Build history of the part. All positions in model axes, mm. Face numbers are marked on the shaded views. Give positions to 0.01 mm unless a question says otherwise; leave off trailing zeros. Order: outer loops, then holes, each group sorted by start corner. A loop starts at its lowest first (then second) coordinate and runs counter-clockwise, first axis right, second up. Notation, with made-up numbers: (62, 73) - (76, 73) arc R13 ccw to (76, 77) - close; hole circle Ø2 at (25, 48.5). An arc over 180 degrees is marked (long way). One line per item, written item: value.
```python
from build123d import *

# Parameters (mm, degrees)
SKETCH1_R                  = 12.5
SKETCH1_R_2                = 4
BOSS_EXTRUDE1_DEPTH        = 29
SKETCH2_R                  = 15
BOSS_EXTRUDE2_DEPTH        = 8
SKETCH3_R                  = 4
CUT_EXTRUDE2_DEPTH         = 43.649736224
F_4_0MM_DOWEL_HOLE1_REACH  = 48.947
F_4_0MM_DOWEL_HOLE1_BORE_R = 2


with BuildPart() as part:
    # Sketch1 → Boss-Extrude1 (new body)
    with BuildSketch(Plane.XY):
        with Locations(Location((0, 0, 0), (0, 0, 180))):
            Circle(SKETCH1_R)
        with Locations(Location((0, 0, 0), (0, 0, 180))):
            Circle(SKETCH1_R_2, mode=Mode.SUBTRACT)
    extrude(amount=BOSS_EXTRUDE1_DEPTH)

    # Sketch2 → Boss-Extrude2 (add)
    with BuildSketch(Plane.XY.offset(29)):
        Circle(SKETCH2_R)
    extrude(amount=BOSS_EXTRUDE2_DEPTH)

    # Sketch3 → Cut-Extrude2 (cut, through all)
    with BuildSketch(Plane(origin=(0, 0, 0), x_dir=(-1, 0, 0), z_dir=(0, 0, -1))):
        Circle(SKETCH3_R)
    extrude(amount=-CUT_EXTRUDE2_DEPTH, mode=Mode.SUBTRACT)

    # Ø4.0mm Dowel Hole1 bore (on position points) → Ø4.0mm Dowel Hole1 (cut, up to next)
    with BuildSketch(Plane(origin=(-14.99999933, 0.004483968, 32.846680342), x_dir=(-0.000298931176, -0.99999995532, 0), z_dir=(-0.99999995532, 0.000298931176, 0)), mode=Mode.PRIVATE) as f_4_0mm_dowel_hole1_sk1:
        Circle(F_4_0MM_DOWEL_HOLE1_BORE_R)
    f_4_0mm_dowel_hole1_tool1 = extrude(f_4_0mm_dowel_hole1_sk1.sketch, amount=-F_4_0MM_DOWEL_HOLE1_REACH, mode=Mode.PRIVATE) & part.part
    add(f_4_0mm_dowel_hole1_tool1.solids().sort_by_distance((-14.999999, 0.004484, 32.84668))[0], mode=Mode.SUBTRACT)


solid = part.part
```
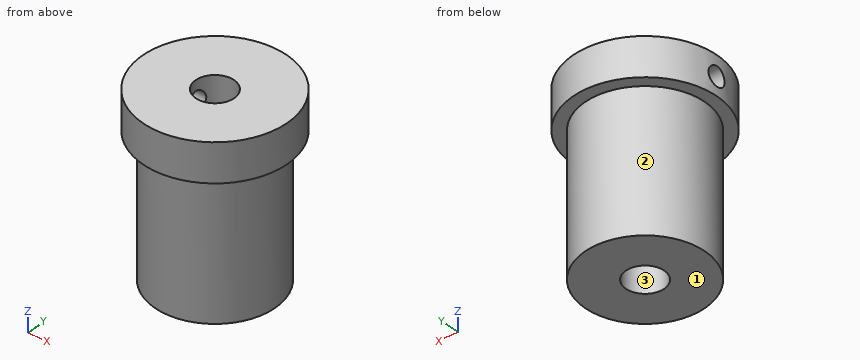
(1) Slice it at D-D, the plane z = 22.5. Give the cut face in (x, y), and give its area (3 significant figures).
Completed:
outline: circle Ø25 at (0, 0); hole circle Ø8 at (0, 0)
area: 441 mm²
(2) Pin check, flat tips, straight feed: P1, Ø1, axis at y = -1, z = 13.5, coming from the -X side; P2, Ø2, axis at x = -1.5, z = 30.5, coming from the -Y side; P3, Ø1, axis at y = -6.5, z = 31, coming from the -X side. Stop position of each tip, or through.
Completed:
P1: x = -12.49
P2: y = -14.99
P3: x = -13.75
(3) Pull direction Y, two halves, no side cores. Call the marked faces 1, 2 and 3: +Y half, -Y half, draft (parallel to the pull), parting line (faces both ways), or undercut.
Completed:
face 1: draft
face 2: parting line
face 3: undercut
(4) Drill centre lines: line 1 (Y direction, x = 0, z = 8.5); line 2 (Z direction, x = -13, y = 5.5); line 3 (X direction, y = -2, z = 16). Where is each one in solid material? Low to high.
Completed:
line 1: -12.5 to -4, 4 to 12.5
line 2: 29 to 37
line 3: -12.34 to -3.46, 3.46 to 12.34
(5) Slice it at C-C, the plane x = 9. Give the cut face in (y, z).
Completed:
outline: (-12, 29) - (-8.67, 29) - (-8.67, 0) - (8.67, 0) - (8.67, 29) - (12, 29) - (12, 37) - (-12, 37) - close
(6) Slice it at A-A, the plane x = 0. Give the cut face in (y, z), and give its area (3 significant figures).
Completed:
outline: (-15, 29) - (-12.5, 29) - (-12.5, 0) - (-4, 0) - (-4, 37) - (-15, 37) - close; (4, 0) - (12.5, 0) - (12.5, 29) - (15, 29) - (15, 37) - (4, 37) - close
area: 669 mm²
(7) Slice it at B-B, the plane y = -3.5. Give the cut face in (x, z), and give its area (3 significant figures).
Completed:
outline: (-14.59, 29) - (-12, 29) - (-12, 0) - (-1.94, 0) - (-1.94, 37) - (-14.59, 37) - close; (1.94, 0) - (12, 0) - (12, 29) - (14.59, 29) - (14.59, 37) - (1.94, 37) - close
area: 786 mm²
